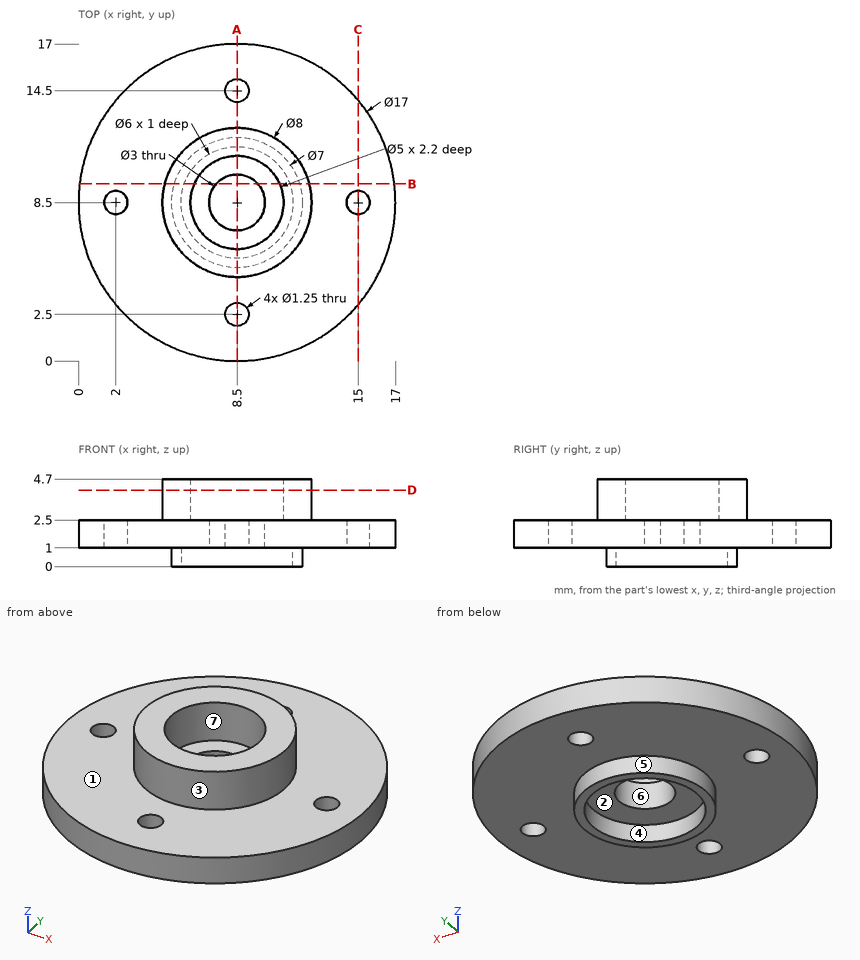
Input: dimensioned drawing with shaded views. Units: mm. Origin: part minimum x, y, z. A direction names the side the tool comes from. Round coordinates to 2 decimals unless told otherwise and drop trailing zeros. Loops run counter-clockwise (first coordinate to the right, second up) from the corner with the lowest first, then second, coordinate; pieces in that order, holes last. Notation, with made-up numbers: (-24.75, 54.25) -> (-2.75, 54.25) arc R19 cw to (-2.75, 79.25) -> close; hole circle Ø11 at (-20, 61.5). An arc over 180 degrees is marked (long way). Use one line per item in the form item = value. Start each with the question number.
1) Section D-D on z = 4.1. Output: boundary loops of the cut face in (x, y), then the cut area to 3 significant figures.
2) First-contact query: P1, Ø3.5, axis at x = 8.5, y = 8.5, coming from the +Z side; P2, Ø1.5, axis at x = 7.5, z = 0.5, coming from the -Y side; P3, Ø1.8, axis at x = 8.5, y = 7, coming from the -Z side. Flat tips, straight axial feed; report the tip coordinate or a pass-through.
3) Section A-A on x = 8.5. Give the number of separate pieces and of enclosed holes in the cut face, then the cut area to 4 significant figures.
4) Draft query along Y for the marked faces 1, 2, 3 and 4. Return one class per face: released by +Y, released by -Y, zero draft, split by the parting line, or undercut.
5) Line query: L1, parallel to Y at x = 8.5, z = 0.45; L2, parallel to Z at x = 7.5, y = 15; L3, parallel to Z at x = 11.5, y = 10.5. Output: solid intervals per line, ascending.
6) Section C-C on x = 15. Output: boundary loops of the cut face in (y, z) (3 decimals), then the cut area to 3 significant figures.
7) Section B-B on y = 9.5. Output: boundary loops of the cut face in (x, z).
8) Access query for the marked faces 5, 6 and 7. Directions: +Z, -Z, +X, -X, +Y, -Y. A direction counts if a zero-diameter tool reaches every point of the face in a straight line with its end or side. Return the directions, or none.
Response:
q1.outline = circle Ø8 at (8.5, 8.5); hole circle Ø5 at (8.5, 8.5)
q1.area = 30.6 mm^2
q2.P1 = 2.5
q2.P2 = 0.01
q2.P3 = 1
q3.separate_pieces = 4
q3.enclosed_holes = 0
q3.area = 24.85 mm^2
q4.face_1 = zero draft
q4.face_2 = undercut
q4.face_3 = split by the parting line
q4.face_4 = undercut
q5.L1 = 5 to 5.5, 11.5 to 12
q5.L2 = 1 to 2.5
q5.L3 = 1 to 4.7
q6.outline = (3.023, 1) -> (7.875, 1) -> (7.875, 2.5) -> (3.023, 2.5) -> close; (9.125, 1) -> (13.977, 1) -> (13.977, 2.5) -> (9.125, 2.5) -> close
q6.area = 14.6 mm^2
q7.outline = (0.06, 1) -> (5.15, 1) -> (5.15, 0) -> (5.67, 0) -> (5.67, 1) -> (7.38, 1) -> (7.38, 2.5) -> (6.21, 2.5) -> (6.21, 4.7) -> (4.63, 4.7) -> (4.63, 2.5) -> (0.06, 2.5) -> close; (9.62, 1) -> (11.33, 1) -> (11.33, 0) -> (11.85, 0) -> (11.85, 1) -> (16.94, 1) -> (16.94, 2.5) -> (12.37, 2.5) -> (12.37, 4.7) -> (10.79, 4.7) -> (10.79, 2.5) -> (9.62, 2.5) -> close
q8.face_5 = -Z
q8.face_6 = +Z, -Z
q8.face_7 = +Z
